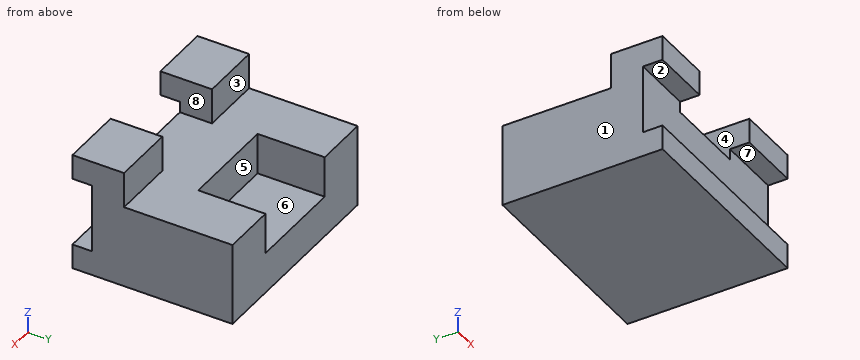
from build123d import *

# Parameters (mm, degrees)
SKETCH1_W               = 254
SKETCH1_H               = 165.1
BOSS_EXTRUDE1_DEPTH     = 101.6
SKETCH2_W               = 120.519823472
SKETCH2_H               = 82.55
CUT_EXTRUDE1_DEPTH      = 50.8
BOSS_EXTRUDE2_DEPTH     = 31.75
CUT_EXTRUDE2_DEPTH      = 315.266796717
CUT_EXTRUDE2_DEPTH_BACK = 315.266796717
SKETCH4_W               = 84.584252786
SKETCH4_H               = 23.924522196


with BuildPart() as part:
    # Sketch1 → Boss-Extrude1 (new body)
    with BuildSketch(Plane.XY):
        Rectangle(SKETCH1_W, SKETCH1_H)
    extrude(amount=BOSS_EXTRUDE1_DEPTH)

    # Sketch2 → Cut-Extrude1 (cut)
    with BuildSketch(Plane.XY.offset(101.6)):
        with Locations((0, 41.275)):
            Rectangle(SKETCH2_W, SKETCH2_H)
    extrude(amount=-CUT_EXTRUDE1_DEPTH, mode=Mode.SUBTRACT)

    # Sketch3 → Boss-Extrude2 (add, symmetric)
    with BuildSketch(Plane(origin=(0, -82.55, 0), x_dir=(-1, 0, 0), z_dir=(0, -1, 0))):
        Polygon((-127, -101.6), (-127, -145.544252786), (-49.406360538, -145.543564589), (-49.406360538, -101.6), (51.702787408, -101.6), (51.702787408, -145.542667829), (127, -145.542), (127, -101.6), (127, 0), (-127, 0), align=None)
    extrude(amount=BOSS_EXTRUDE2_DEPTH, both=True)

    # Sketch4 → Cut-Extrude2 (cut, two sides: drawn at the far end of the back side and taken through both)
    with BuildSketch(Plane(origin=(127, 0, 0), x_dir=(0, 0, -1), z_dir=(1, 0, 0)).offset(-CUT_EXTRUDE2_DEPTH_BACK)):
        with Locations((-72.772126393, -102.337738902)):
            Rectangle(SKETCH4_W, SKETCH4_H)
    extrude(amount=CUT_EXTRUDE2_DEPTH + CUT_EXTRUDE2_DEPTH_BACK, mode=Mode.SUBTRACT)


solid = part.part
Part model, mm, in its own coordinate system. Face numbers are marked on the shaded views. A direction names the side the tool comes from. Round coordinates to 2 decimals unless told otherwise and drop trailing zeros. Write each loop counter-clockwise with the first axis right and the second up, starting at its lowest first coordinate (ties: lowest second). Pieces come first, ordered by that corner, then holes. Notation, with made-up numbers: M -39,-10 L 20,-10 A19 cw 20,15 Z; hole C 23.5,-33 d7. An arc over 180 degrees is marked long. Return JSON: item names as keys, results as strings. Group by question number.
(1) Drill centre lines: probe 1 along Z at (x, y) = (67, -91.5); probe 2 along X at (y, z) = (36, 60); probe 3 along Z at (x, y) = (-18.5, 42). Where is each one in solid material? Low to high.
(2) Saw through at C-C on z = 124. Write the cut outline in (x, y), then the cut area to 3 significant figures.
(3) Saw through at D-D on x = -104.5. Write the cut outline in (y, z), then the cut area to 3 significant figures.
(4) Saw through at B-B on y = 45. Write the cut outline in (x, z), then the cut area to 3 significant figures.
(5) Pin check, flat tips, straight feed: pin 1 Ø13 at (x, z) = (-73, 120) entering from +Y; pin 2 Ø12 at (x, z) = (-21, 99.5) entering from -Y; pin 3 Ø2 at (x, y) = (-45.5, 28.5) entering from +Z. Stop position of each tip, or through.
(6) Which spindle directions (+Z, -Z, +X, -X, +Y, -Y) get a long thin tool onto all of the face, cutting with end or side? Do the marked faces 1, 2, 3, 4 and 5. Say none if no direction does.
(7) Two-plate mould, pull along Z, no slides. Class the marked faces 6, 7 and 8: +Z half, -Z half, draft (parallel to the pull), parting line (faces both ways), or undercut.
(8) Saw through at A-A on z = 79. Write the cut outline in (x, y), then the cut area to 3 significant figures.
Returned:
{
 "1": {"probe 1": "0 to 30.48, 115.06 to 145.54", "probe 2": "-127 to -60.26, 60.26 to 127", "probe 3": "0 to 50.8"},
 "2": {"outline": "M -127,-114.3 L -51.7,-114.3 L -51.7,-50.8 L -127,-50.8 Z; M 49.41,-114.3 L 127,-114.3 L 127,-50.8 L 49.41,-50.8 Z", "area": "9,710 mm²"},
 "3": {"outline": "M -114.3,0 L 82.55,0 L 82.55,101.6 L -50.8,101.6 L -50.8,145.54 L -114.3,145.54 L -114.3,115.06 L -90.38,115.06 L -90.38,30.48 L -114.3,30.48 Z", "area": "20,800 mm²"},
 "4": {"outline": "M -127,0 L 127,0 L 127,101.6 L 60.26,101.6 L 60.26,50.8 L -60.26,50.8 L -60.26,101.6 L -127,101.6 Z", "area": "19,700 mm²"},
 "5": {"pin 1": "y = -50.8", "pin 2": "y = -90.38", "pin 3": "z = 50.8"},
 "6": {"face 1": "+Z, -Z, -X, +Y, -Y", "face 2": "+X, -X, -Y", "face 3": "+Z, +X, -X, +Y", "face 4": "+Z, +Y, -Y", "face 5": "+Z, +Y"},
 "7": {"face 6": "+Z half", "face 7": "undercut", "face 8": "draft"},
 "8": {"outline": "M -127,-90.38 L 127,-90.38 L 127,82.55 L 60.26,82.55 L 60.26,0 L -60.26,0 L -60.26,82.55 L -127,82.55 Z", "area": "34,000 mm²"}
}
